Design review of the part built by this model. Coordinates are the model's own, in mm. A direction names the side the tool comes from. Give positions to 0.01 mm unless a question says otherwise; leave off trailing zeros. Loops run counter-clockwise (first coordinate to the right, second up) from the corner with the lowest first, then second, coordinate; pieces in that order, holes last. Notation, with made-up numbers: (18.25, 72.5) - (52.25, 72.5) arc R34 cw to (52.25, 111.5) - close; hole circle Ø1 at (-9, -31.75). An arc over 180 degrees is marked (long way). Put each result on its own line as item: value. Start each with the question number.
```python
from build123d import *

# Parameters (mm, degrees)
F0_W     = 25.4
F0_H     = 25.4
F0_W_2   = 22.225
F0_H_2   = 22.225
F1_DEPTH = 548.64
F3_DEPTH = 25.401
F5_DEPTH = 25.401


with BuildPart() as f1:
    # F0 (on Front) → F1 (new body, symmetric)
    with BuildSketch(Plane.XZ):
        Rectangle(F0_W, F0_H)
        Rectangle(F0_W_2, F0_H_2, mode=Mode.SUBTRACT)
    extrude(amount=F1_DEPTH, both=True)

    # F2 (on face) → F3 (cut, through all)
    with BuildSketch(Plane.XY.offset(12.7)):
        Polygon((12.7, 548.64), (-12.7, 548.64), (-12.7, 541.691346), align=None)
    extrude(amount=-F3_DEPTH, mode=Mode.SUBTRACT)

    # F4 (on face) → F5 (cut, through all)
    with BuildSketch(Plane.XY.offset(12.7)):
        Polygon((12.7, -541.691346), (-12.7, -548.64), (12.7, -548.64), align=None)
    extrude(amount=-F5_DEPTH, mode=Mode.SUBTRACT)


solid = f1.part
```
Item 1: For P1, Ø6, axis at x = 4, z = -8.5, coming from the -Y side, flat-tipped, find the tip position at first contact; note if it passes through.
Item 2: Mouldability with a two-part tool opening along Z and no side actions: class faces 3 (the flat face through (0, -8, -12.7)), 4 (the flat face through (-11.112, -11, 0)), 5 (the flat face through (0.06, -545.15, 11.35)) as pulls with the +Z half, pulls with the -Z half, needs draft (parallel to the pull), parting line crosses it, or undercut.
Item 3: For L1, parallel to Z at x = 11, y = 302.5, list the stretches that pass through material, from the lowest coordinate up. Write a range as from..to.
Item 4: Consider section C-C (y = -386). State the section outline as (x, z) points, plus the area to 3 significant figures.
Item 5: Machinability: for faces 1 (the flat face through (0, -8, 11.112)), 2 (the flat face through (-0.06, 545.15, 11.35)), which of the approach directions +Z, -Z, +X, -X, +Y, -Y give a long, thin tool a straight path to every point of the face, cutting with its end or side? Answer none if there is none.
Item 6: Consider section A-A (z = -1). State the section outline as (x, y) points.
Item 7: Consider section B-B (x = -3). State the section outline as (y, z) points.
Geometry says:
1. P1: stops at y = -544.47
2. face 3: pulls with the -Z half
2. face 4: undercut
2. face 5: needs draft
3. L1: z = -12.7..-11.11, 11.11..12.7
4. outline: (-12.7, -12.7) - (12.7, -12.7) - (12.7, 12.7) - (-12.7, 12.7) - close; hole (-11.11, -11.11) - (11.11, -11.11) - (11.11, 11.11) - (-11.11, 11.11) - close
4. area: 151 mm2
5. face 1: +Y, -Y
5. face 2: +Z, -Z, -X, +Y
6. outline: (-12.7, -548.64) - (-11.11, -548.21) - (-11.11, 542.13) - (-12.7, 541.69) - close; (11.11, -542.13) - (12.7, -541.69) - (12.7, 548.64) - (11.11, 548.21) - close
7. outline: (-545.99, -12.7) - (544.34, -12.7) - (544.34, -11.11) - (-545.99, -11.11) - close; (-545.99, 11.11) - (544.34, 11.11) - (544.34, 12.7) - (-545.99, 12.7) - close
